from build123d import *

# Parameters (mm, degrees)
SKETCH2_R          = 12.718
CUT_EXTRUDE1_DEPTH = 82.74
SKETCH3_R          = 10
CUT_EXTRUDE2_DEPTH = 79.507
SKETCH4_W          = 1.691
SKETCH4_H          = 6.375
CUT_EXTRUDE3_DEPTH = 56


with BuildPart() as part:
    # Sketch1 → Revolve1 (revolve)
    with BuildSketch(Plane.XY, mode=Mode.PRIVATE) as revolve1_sk:
        with BuildLine():
            Line((-80.911998208, 0), (-80.911998208, 12.718))
            Line((-80.911998208, 12.718), (-70.911998208, 12.718))
            Line((-70.911998208, 12.718), (-70.911998208, 32.718))
            add(Edge.make_bspline(
                [(-70.911998208, 32.718), (-72.12061009, 49.624927681), (-53.086599537, 70.223127666), (-24.900561644, 82.171389104), (-2.569366769, 92.818520506), (6.899070449, 82.616568551), (10.881080371, 90)],
                knots=[0, 0, 0, 0, 0.424565584, 0.683651406, 0.890381035, 1, 1, 1, 1], degree=3))
            Line((10.881080371, 90), (14.335001792, 90))
            Line((14.335001792, 90), (14.335001792, 93))
            Line((14.335001792, 93), (20.335001792, 93))
            Line((20.335001792, 93), (41.227154337, 15))
            Line((41.227154337, 15), (53.870153491, 15))
            Line((53.870153491, 15), (64.335001792, 91.202154094))
            Line((64.335001792, 91.202154094), (74.335001792, 91.202154094))
            Line((74.335001792, 91.202154094), (74.335001792, 14.709294291))
            Line((74.335001792, 14.709294291), (79.335001792, 14.709294291))
            Line((79.335001792, 14.709294291), (79.335001792, 0))
            Line((79.335001792, 0), (-80.911998208, 0))
        make_face()
    revolve(revolve1_sk.sketch.rotate(Axis((-81.835688806, 0, 0), (1, 0, 0)), 90), axis=Axis((-81.835688806, 0, 0), (1, 0, 0)))

    # Sketch2 → Cut-Extrude1 (cut)
    with BuildSketch(Plane(origin=(79.335001792, 0, 0), x_dir=(0, 0, -1), z_dir=(1, 0, 0))):
        with Locations(Location((0, 0, 0), (0, 0, 180))):
            Circle(SKETCH2_R)
    extrude(amount=-CUT_EXTRUDE1_DEPTH, mode=Mode.SUBTRACT)

    # Sketch3 → Cut-Extrude2 (cut)
    with BuildSketch(Plane.ZY.offset(80.911998208)):
        Circle(SKETCH3_R)
    extrude(amount=-CUT_EXTRUDE2_DEPTH, mode=Mode.SUBTRACT)

    # Chamfer1
    # the kernel refuses this chamfer: 3, 1.732050808 mm, written as the material it takes off along each edge
    with BuildSketch(Plane(origin=(-3.404998208, 0, 0), x_dir=(0, 0, 1), z_dir=(0, -1, 0))) as chamfer1_piece_1_section:
        with BuildLine():
            Line((9.896076952, 1.792050808), (13.103923048, -0.06))
            Line((13.103923048, -0.06), (13.103923048, -0.12))
            ThreePointArc((13.103923048, -0.12), (11.551961524, -0.06), (10, -0.06))
            Line((10, -0.06), (9.94, 0))
            ThreePointArc((9.94, 0), (9.94, 0.896025404), (9.836076952, 1.792050808))
            Line((9.836076952, 1.792050808), (9.896076952, 1.792050808))
        make_face()
    chamfer1_piece_1 = revolve(axis=Axis((-3.404998208, 0, 0), (-1, 0, 0)), mode=Mode.PRIVATE)
    chamfer1_piece_1 = chamfer1_piece_1 & Plane(origin=(-4.331873762, 0, 0), x_dir=(0, 0, 1), z_dir=(1, 0, 0)) * Cylinder(12.718, 53, mode=Mode.PRIVATE)
    add(chamfer1_piece_1, mode=Mode.SUBTRACT)

    # Sketch4 → Cut-Extrude3 (cut)
    with BuildSketch(Plane(origin=(79.335001792, 0, 0), x_dir=(0, 0, -1), z_dir=(1, 0, 0))):
        with Locations((12.718, 0)):
            Rectangle(SKETCH4_W, SKETCH4_H)
    extrude(amount=-CUT_EXTRUDE3_DEPTH, mode=Mode.SUBTRACT)


solid = part.part
Input: part model. Units: mm. Frame: model coordinates. A direction names the side the tool comes from. Give positions to 0.01 mm unless a question says otherwise; leave off trailing zeros. Write item = value, one per line. Start each with the question number.
1) First-contact query: pin 1 Ø1 at (y, z) = (-29, 13.5) entering from -X; pin 2 Ø3 at (x, y) = (-40.5, -46.5) entering from +Z; pin 3 Ø12 at (x, z) = (-25.5, 28.5) entering from +Y. Flat tips, straight axial feed; report the tip coordinate or a pass-through.
2) Reachability of faces 1 (the cylindrical face through (47.64, -12.65, 8.06)), 2 (the flat face through (52, 0, -13.564)), 3 (the flat face through (-70.912, 14, 0)), 4 (the cylindrical face through (-43.55, 3, 9.54)) from +Z, -Z, +X, -X, +Y, -Y: full face, straight path, thin tool, end or side. Return the list, or none.
3) Material intervals for line 1 along Y through (x, z) = (43, 0); line 2 along X through (y, z) = (30.5, 81) (3 decimals); line 3 along X through (y, z) = (-78, 1) (1 decimal), sorted ascending. Write a range as [from, to].
4) Draft query along Y for faces 5 (the flat face through (-80.912, 7, 8)), 6 (the conical face through (54.525, -5.937, 18.854)), 7 (the conical face through (-5.04, 3.05, 9.7)). Return one class per face: +Y half, -Y half, draft (parallel to the pull), parting line (faces both ways), or undercut.
Solved:
q1.pin_1 = -70.91
q1.pin_2 = 60.29
q1.pin_3 = 80.54
q2.face_1 = none
q2.face_2 = +X
q2.face_3 = -X
q2.face_4 = +X, -X
q3.line_1 = [-15, -12.72], [12.72, 15]
q3.line_2 = [-15.47, 2.356], [8.316, 22.062], [63.696, 74.335]
q3.line_3 = [-34.4, 24.4], [62.5, 74.3]
q4.face_5 = draft
q4.face_6 = parting line
q4.face_7 = undercut
